Autodesk Inventor part; units mm, degrees
ref_plane "YZ Plane" through (0, 0, 0) normal (1, 0, 0) x (0, 1, 0)
ref_plane "XZ Plane" through (0, 0, 0) normal (0, 1, 0) x (-1, 0, 0)
ref_plane "XY Plane" through (0, 0, 0) normal (0, 0, 1) x (1, 0, 0)
sketch "Sketch1" plane through (0, 0, 0) normal (0, 0, 1) x (1, 0, 0)
  circle A0 centre (10.6405, 2.5912) radius 4
  line L0 (15.6405, 6.5912) -> (5.6405, 6.5912)
  line L1 (4.6405, 5.5912) -> (4.6405, -0.4088)
  line L2 (5.6405, -1.4088) -> (15.6405, -1.4088)
  line L3 (16.6405, -0.4088) -> (16.6405, 5.5912)
  line L4 (16.6405, 6.5912) -> (4.6405, -1.4088) construction
  line L5 (4.6405, 6.5912) -> (16.6405, -1.4088) construction
  arc A1 (5.6405, 6.5912) -> (4.6405, 5.5912) centre (5.6405, 5.5912) ccw
  arc A2 (4.6405, -0.4088) -> (5.6405, -1.4088) centre (5.6405, -0.4088) ccw
  arc A3 (15.6405, -1.4088) -> (16.6405, -0.4088) centre (15.6405, -0.4088) ccw
  arc A4 (16.6405, 5.5912) -> (15.6405, 6.5912) centre (15.6405, 5.5912) ccw
  point P0 (0, 0)
  point P1 (10.6405, 6.5912)
  point P2 (10.6405, -1.4088)
  dimension "d6" = 8
  dimension "d13" = 8
  dimension "d14" = 12
  dimension "d15" = 1
extrude "Extrusion1" add sketch "Sketch1" along normal blind 1
sketch "Sketch2" plane through (10.6405, 2.5912, 0) normal (0, 0, -1) x (-1, 0, 0)
  circle A0 centre (0, 0) radius 3
  line L0 (5, -4) -> (-5, -4)
  arc A1 (-6, -3) -> (-5, -4) centre (-5, -3) ccw
  line L1 (-6, -3) -> (-6, 3)
  arc A2 (-5, 4) -> (-6, 3) centre (-5, 3) ccw
  line L2 (-5, 4) -> (5, 4)
  arc A3 (6, 3) -> (5, 4) centre (5, 3) ccw
  line L3 (6, 3) -> (6, -3)
  arc A4 (5, -4) -> (6, -3) centre (5, -3) ccw
  line L4 (-4, -3) -> (4, -3)
  line L5 (5, -2) -> (5, 2)
  line L6 (4, 3) -> (-4, 3)
  line L7 (-5, 2) -> (-5, -2)
  arc A5 (5, 2) -> (4, 3) centre (4, 2) ccw
  arc A6 (4, -3) -> (5, -2) centre (4, -2) ccw
  arc A7 (-5, -2) -> (-4, -3) centre (-4, -2) ccw
  arc A8 (-4, 3) -> (-5, 2) centre (-4, 2) ccw
  point P0 (10.6405, -2.5912)
  point P1 (0, 3)
  point P2 (0, -3)
  dimension "d16" = 1
  dimension "d17" = 1
extrude "Extrusion2" add sketch "Sketch2" along normal blind 1.3 and the other way blind 3.5 contours A0 | A0 L6 A5 L5 A6 L4 | A0 L4 A7 L7 A8 L6
fillet "Fillet3" radius 0.5 10 edges at (15.3476, -0.1159, 3.5) (15.6405, 2.5912, 3.5) (15.3476, 5.2983, 3.5) (12.6405, 5.5912, 3.5) (8.6405, 5.5912, 3.5) (5.9334, 5.2983, 3.5) (5.6405, 2.5912, 3.5) (5.9334, -0.1159, 3.5) (8.6405, -0.4088, 3.5) (12.6405, -0.4088, 3.5)
sketch "Sketch4" plane through (0, 0, 0) normal (0, 0, -1) x (-1, 0, 0)
  point P0 (0, 0)
sketch "Sketch6" plane through (0, 0, 0) normal (0, 0, -1) x (-1, 0, 0)
  arc A0 (-15.6405, 0.5912) -> (-14.6405, -0.4088) centre (-14.6405, 0.5912) ccw
  line L0 (-15.6405, 0.5912) -> (-15.6405, 4.5912)
  arc A1 (-14.6405, 5.5912) -> (-15.6405, 4.5912) centre (-14.6405, 4.5912) ccw
  line L1 (-14.6405, 5.5912) -> (-6.6405, 5.5912)
  arc A2 (-5.6405, 4.5912) -> (-6.6405, 5.5912) centre (-6.6405, 4.5912) ccw
  line L2 (-5.6405, 4.5912) -> (-5.6405, 0.5912)
  arc A3 (-6.6405, -0.4088) -> (-5.6405, 0.5912) centre (-6.6405, 0.5912) ccw
  line L3 (-6.6405, -0.4088) -> (-14.6405, -0.4088)
  line L4 (-5.6405, -1.4088) -> (-15.6405, -1.4088)
  arc A4 (-5.6405, -1.4088) -> (-4.6405, -0.4088) centre (-5.6405, -0.4088) ccw
  line L5 (-4.6405, 5.5912) -> (-4.6405, -0.4088)
  arc A5 (-4.6405, 5.5912) -> (-5.6405, 6.5912) centre (-5.6405, 5.5912) ccw
  line L6 (-15.6405, 6.5912) -> (-5.6405, 6.5912)
  arc A6 (-15.6405, 6.5912) -> (-16.6405, 5.5912) centre (-15.6405, 5.5912) ccw
  line L7 (-16.6405, -0.4088) -> (-16.6405, 5.5912)
  arc A7 (-16.6405, -0.4088) -> (-15.6405, -1.4088) centre (-15.6405, -0.4088) ccw
  point P0 (0, 0)
extrude "Extrusion5" add sketch "Sketch6" along normal up to surface (1.3 mm away)
sketch "Sketch7" plane through (10.6405, 2.5912, -1.3) normal (0, 0, -1) x (-1, 0, 0)
  arc A0 (6, 3) -> (5, 4) centre (5, 3) ccw
  line L0 (-5, 4) -> (5, 4)
  arc A1 (-5, 4) -> (-6, 3) centre (-5, 3) ccw
  line L1 (-6, -3) -> (-6, 3)
  arc A2 (-6, -3) -> (-5, -4) centre (-5, -3) ccw
  line L2 (5, -4) -> (-5, -4)
  arc A3 (5, -4) -> (6, -3) centre (5, -3) ccw
  line L3 (6, 3) -> (6, -3)
  line L4 (4, -2) -> (-4, -2)
  line L5 (-4, -2) -> (-4, 2)
  line L6 (-4, 2) -> (4, 2)
  line L7 (4, 2) -> (4, -2)
  point P0 (10.6405, -2.5912)
  dimension "d28" = 2
extrude "Extrusion6" cut sketch "Sketch7" against normal blind 1.5
chamfer "Chamfer2" distance 1.5 angle 45 4 edges at (10.6405, 0.5912, 0.2) (6.6405, 2.5912, 0.2) (10.6405, 4.5912, 0.2) (14.6405, 2.5912, 0.2)
properties part number "button_3DPrint"
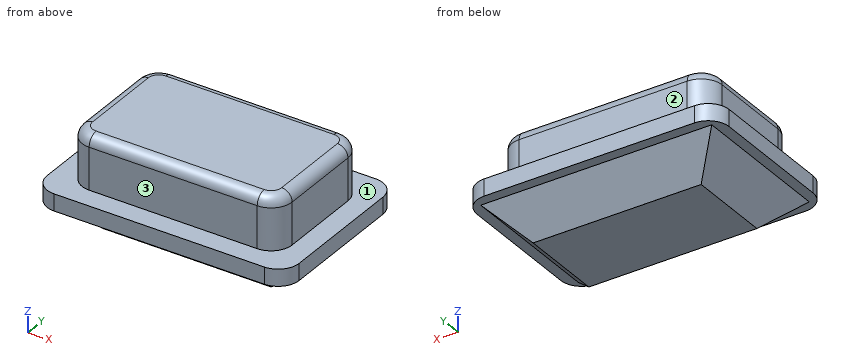
Part model, mm, in its own coordinate system. Face numbers are marked on the shaded views. A direction names the side the tool comes from. Give positions to 0.01 mm unless a question says otherwise; leave off trailing zeros. Loops run counter-clockwise (first coordinate to the right, second up) from the corner with the lowest first, then second, coordinate; pieces in that order, holes last.
(1) Band-saw the part on D-D (z = -0.05). Write the cut outline in (x, y), and give its area (3 significant figures).
Return value:
outline: (5.39, -0.66) - (15.89, -0.66) - (15.89, 5.84) - (5.39, 5.84) - close
area: 68.2 mm2
(2) 3-axis set-ups, long thin cutter, end or side, ignore diameter. For the marked faces 1, 2 and 3: which of +Z, -Z, +X, -X, +Y, -Y reach the whole face in a straight line?
Return value:
face 1: +Z
face 2: +Z, +X, -X, +Y
face 3: +Z, +X, -X, -Y
(3) Drill centre lines: line 1 along X through (y, z) = (3, -0.8); line 2 along X through (y, z) = (3, 2.3); line 3 along Y through (x, z) = (7.75, 2.85). Where is each one in solid material? Low to high.
Return value:
line 1: x = 6.14 to 15.14
line 2: x = 5.64 to 15.64
line 3: y = -0.41 to 5.59
(4) Pin check, flat tips, straight feed: pin 1 (1.5 mm diameter, centred on x = 6.5, z = 3, fed in from +Y); pin 2 (0.6 mm diameter, centred on y = 2.5, z = 2.5, fed in from -X); pin 3 (0.6 mm diameter, centred on y = 2, z = 2, fed in from +X); pin 4 (4 mm diameter, centred on x = 6.5, y = 5, fed in from -Z). Stop position of each tip, or through.
Return value:
pin 1: stops at y = 5.59
pin 2: stops at x = 5.64
pin 3: stops at x = 15.64
pin 4: stops at z = -1.3
(5) Band-saw the part on C-C (z = 2.75). Write the cut outline in (x, y).
Return value:
outline: (5.64, 0.59) arc R1 ccw to (6.64, -0.41) - (14.64, -0.41) arc R1 ccw to (15.64, 0.59) - (15.64, 4.59) arc R1 ccw to (14.64, 5.59) - (6.64, 5.59) arc R1 ccw to (5.64, 4.59) - close
